```python
from build123d import *

# Parameters (mm, degrees)
CROQUIS1_W              = 1.314474999
CROQUIS1_H              = 9.624843278
SALIENTE_EXTRUIR1_DEPTH = 7
SALIENTE_EXTRUIR2_DEPTH = 10.19818
CROQUIS3_R              = 2.216125171
CORTAR_EXTRUIR1_DEPTH   = 10
CROQUIS4_R              = 0.491522535
SALIENTE_EXTRUIR3_DEPTH = 8
REDONDEO1_R             = 0.2
SALIENTE_EXTRUIR4_DEPTH = 0.5


with BuildPart() as part:
    # Croquis1 → Saliente-Extruir1 (new body)
    with BuildSketch(Plane(origin=(0, 31.468175746, 0), x_dir=(1, 0, 0), z_dir=(0, 1, 0))):
        with Locations((-13.550232167, -69.22627342)):
            Rectangle(CROQUIS1_W, CROQUIS1_H)
    extrude(amount=SALIENTE_EXTRUIR1_DEPTH)

    # Croquis2 → Saliente-Extruir2 (add)
    with BuildSketch(Plane(origin=(-12.892994667, 0, 0), x_dir=(0, 0, -1), z_dir=(1, 0, 0))):
        with BuildLine():
            ThreePointArc((-73.620597099, 31.468175746), (-73.933010103, 32.427133129), (-74.038695059, 33.430144513))
            Line((-74.038695059, 33.430144513), (-74.038695059, 31.468175746))
            Line((-74.038695059, 31.468175746), (-73.620597099, 31.468175746))
        make_face()
        with BuildLine():
            Line((-64.413851781, 31.468175746), (-64.413851781, 33.430144513))
            ThreePointArc((-64.413851781, 33.430144513), (-64.519536737, 32.427133129), (-64.831949741, 31.468175746))
            Line((-64.831949741, 31.468175746), (-64.413851781, 31.468175746))
        make_face()
        with BuildLine():
            ThreePointArc((-64.831949741, 31.468175746), (-64.519536737, 32.427133129), (-64.413851781, 33.430144513))
            ThreePointArc((-64.413851781, 33.430144513), (-69.22627342, 38.242566152), (-74.038695059, 33.430144513))
            ThreePointArc((-74.038695059, 33.430144513), (-73.933010103, 32.427133129), (-73.620597099, 31.468175746))
            Line((-73.620597099, 31.468175746), (-64.831949741, 31.468175746))
        make_face()
    extrude(amount=SALIENTE_EXTRUIR2_DEPTH)

    # Croquis3 → Cortar-Extruir1 (cut)
    with BuildSketch(Plane.ZY.offset(14.207469666)):
        with Locations((69.22627342, 35.266765238)):
            Circle(CROQUIS3_R)
    extrude(amount=-CORTAR_EXTRUIR1_DEPTH, mode=Mode.SUBTRACT)

    # Croquis4 → Saliente-Extruir3 (add)
    with BuildSketch(Plane.ZY.offset(4.207469666)):
        with Locations((69.22627342, 35.266765238)):
            Circle(CROQUIS4_R)
    extrude(amount=SALIENTE_EXTRUIR3_DEPTH)

    # Redondeo1
    redondeo1_edges = [part.edges().sort_by_distance(p)[0] for p in [
        (-12.207469666, 35.266765238, 68.734750885),
    ]]
    fillet(redondeo1_edges, radius=REDONDEO1_R)

    # Croquis5 → Saliente-Extruir4 (add)
    with BuildSketch(Plane(origin=(-2.694814404, 0, 0), x_dir=(0, 0, -1), z_dir=(1, 0, 0))):
        with BuildLine():
            Line((-70.108064563, 36.024784092), (-70.108064563, 32.468175746))
            Line((-70.108064563, 32.468175746), (-68.344482277, 32.468175746))
            Line((-68.344482277, 32.468175746), (-68.344482277, 36.024784092))
            ThreePointArc((-68.344482277, 36.024784092), (-69.22627342, 36.906575235), (-70.108064563, 36.024784092))
        make_face()
    extrude(amount=SALIENTE_EXTRUIR4_DEPTH)


solid = part.part
```
For this review, take the finished solid that the model builds, in its own axes (mm). A direction names the side the tool comes from. Coordinates: 2 decimals unless noted, no trailing zeros. Loops run counter-clockwise (first coordinate to the right, second up) from the corner with the lowest first, then second, coordinate; pieces in that order, holes last.
1. For line 1 (Y direction, x = -5, z = 69); line 2 (X direction, y = 34.25, z = 68); line 3 (X direction, y = 35.5, z = 65.25), list the stretches that pass through material, from the lowest coordinate up.
2. Insertion check: P1, Ø1, axis at y = 37, z = 73, coming from the +X side; P2, Ø1, axis at x = -6.5, z = 72.5, coming from the +Y side. Each pin has a flat end and moves straight along its axis. Give the tip position at first contact, or say it passes through.
3. For faces 1 (the cylindrical face through (-8.05, 34.83, 69.45)), 2 (the cylindrical face through (-2.448, 36.906, 69.207)), 3 (the flat face through (-10, 33, 64.414)), list the 3-axis set-ups (+Z, -Z, +X, -X, +Y, -Y) from which the entire face can be reached by the end or side of a thin tool; tool diameter is ignored.
4. Add section C-C, the plane z = 65. Give the boundary of the cut face in (x, y), then the cut area to 3 significant figures.
5. Add section A-A, the plane x = -5.75. Give the boundary of the cut face in (y, z).
6. Mouldability with a two-part tool opening along Y and no side actions: class faces 4 (the flat face through (-14, 38.468, 69)), 5 (the flat face through (-12.893, 38.2, 67.8)), 6 (the flat face through (-4.207, 36, 69)) as +Y half, -Y half, draft (parallel to the pull), parting line (faces both ways), or undercut.
7. Add section D-D, the plane x = -3. Give the boundary of the cut face in (y, z), then the cut area to 3 significant figures.
8. Add section B-B, the plane y = 38. Give the boundary of the cut face in (x, z), then the cut area to 3 significant figures.
Result:
1. line 1: y = 31.47 to 33.06, 34.83 to 35.7, 37.47 to 38.24
1. line 2: x = -4.21 to -2.69
1. line 3: x = -14.21 to -2.69
2. P1: stops at x = -2.69
2. P2: stops at y = 37.36
3. face 1: -X
3. face 2: +X, +Y
3. face 3: -Z, +X, -X, +Y, -Y
4. outline: (-14.21, 31.47) - (-2.69, 31.47) - (-2.69, 35.73) - (-12.89, 35.73) - (-12.89, 38.47) - (-14.21, 38.47) - close
4. area: 52.7 mm2
5. outline: (31.47, 64.41) - (33.43, 64.41) arc R4.81 ccw to (33.43, 74.04) - (31.47, 74.04) - close; circle Ø0.98 at (35.27, 69.23); hole circle Ø4.43 at (35.27, 69.23)
6. face 4: +Y half
6. face 5: draft
6. face 6: undercut
7. outline: (31.47, 64.41) - (33.43, 64.41) arc R4.81 ccw to (33.43, 74.04) - (31.47, 74.04) - close
7. area: 55.3 mm2
8. outline: (-14.21, 64.41) - (-12.89, 64.41) - (-12.89, 67.72) - (-2.69, 67.72) - (-2.69, 70.73) - (-12.89, 70.73) - (-12.89, 74.04) - (-14.21, 74.04) - close
8. area: 43.4 mm2
